```python
from build123d import *

# Parameters (mm, degrees)
F0_R     = 20
F0_R_2   = 9.5
F1_DEPTH = 50
F2_R     = 10
F3_DEPTH = 25
F5_D     = 5
F5_DEPTH = 50
F5_TIP   = 1.5021515476
F7_D     = 5
F7_DEPTH = 50
F7_TIP   = 1.5021515476
F8_R     = 1


with BuildPart() as f1:
    # F0 (on Front) → F1 (new body)
    with BuildSketch(Plane.XZ):
        Circle(F0_R)
        Circle(F0_R_2, mode=Mode.SUBTRACT)
    extrude(amount=F1_DEPTH)

    # F2 (on face) → F3 (cut)
    with BuildSketch(Plane.XZ.offset(50)):
        Circle(F2_R)
    extrude(amount=-F3_DEPTH, mode=Mode.SUBTRACT)

    # F5 (one way)
    with BuildSketch(Plane.YZ):
        with Locations((-42, 0), (-32, 0), (-18, 0), (-8, 0)):
            Circle(F5_D / 2)
    extrude(amount=-F5_DEPTH, mode=Mode.SUBTRACT)
    with Locations(Plane.YZ):
        with Locations((-42, 0), (-32, 0), (-18, 0), (-8, 0)):
            with Locations((0, 0, -(F5_DEPTH + F5_TIP / 2))):  # 118° drill point
                Cone(0, F5_D / 2, F5_TIP, mode=Mode.SUBTRACT)

    # F7 (one way)
    with BuildSketch(Plane.XY):
        with Locations((0, -8), (0, -18), (0, -32), (0, -42)):
            Circle(F7_D / 2)
    extrude(amount=-F7_DEPTH, mode=Mode.SUBTRACT)
    with Locations(Plane.XY):
        with Locations((0, -8), (0, -18), (0, -32), (0, -42)):
            with Locations((0, 0, -(F7_DEPTH + F7_TIP / 2))):  # 118° drill point
                Cone(0, F7_D / 2, F7_TIP, mode=Mode.SUBTRACT)

    # F8
    f8_edges = [f1.edges().sort_by_distance(p)[0] for p in [
        (-9.5, 0, 0),
        (-10, -50, 0),
    ]]
    fillet(f8_edges, radius=F8_R)


solid = f1.part
```
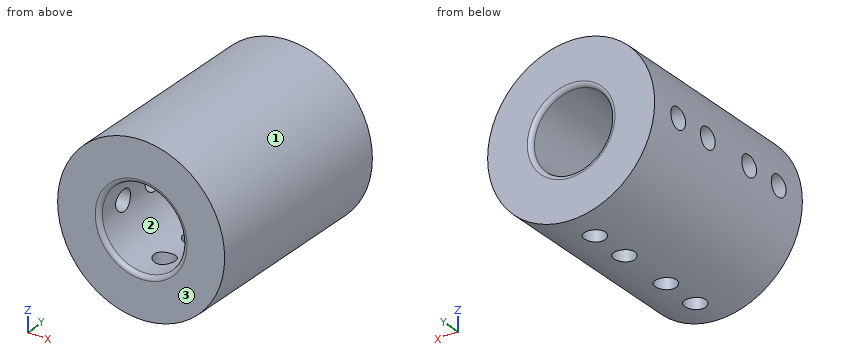
Input: part model. Units: mm. Frame: model coordinates. Face numbers are marked on the shaded views. Give positions to 0.01 mm unless a question says otherwise; leave off trailing zeros. Loops run counter-clockwise (first coordinate to the right, second up) from the corner with the lowest first, then second, coordinate; pieces in that order, holes last.
1) Section query D-D on x = -16. Return the cut outline in (y, z).
A:
outline: (-50, -12) - (0, -12) - (0, 12) - (-50, 12) - close; hole circle Ø5 at (-42, 0); hole circle Ø5 at (-32, 0); hole circle Ø5 at (-18, 0); hole circle Ø5 at (-8, 0)
2) Section query A-A on x = 0. Count the separate pieces of the cut face and the enclosed holes in it, and give its area (3 significant figures).
A:
separate pieces: 6
enclosed holes: 0
area: 819 mm2
3) Section query C-C on y = -8. Return the cut outline in (x, z).
A:
outline: (-19.84, -2.5) arc R20 ccw to (-2.5, -19.84) - (-2.5, -9.17) arc R9.5 cw to (-9.17, -2.5) - close; (-19.84, 2.5) - (-9.17, 2.5) arc R9.5 cw (long way) to (2.5, -9.17) - (2.5, -19.84) arc R20 ccw (long way) to start
4) Contact query for flat-ended pins moving along their axis: pin 1 (8 mm diameter, centred on y = -29, z = 10, fed in from -X); pin 2 (3 mm diameter, centred on y = -11.5, z = 2, fed in from +X); pin 3 (4 mm diameter, centred on x = 0, y = -32, fed in from +Z). Output: stop coordinate, or through.
A:
pin 1: stops at x = -19.08
pin 2: stops at x = 19.99
pin 3: stops at z = 20
5) Line query: L1, parallel to Y at x = 0, z = -15; L2, parallel to X at y = -38.5, z = 0; L3, parallel to Z at x = 0.5, y = -15. Output: solid intervals per line, ascending.
A:
L1: y = -50 to -44.5, -39.5 to -34.5, -29.5 to -20.5, -15.5 to -10.5, -5.5 to 0
L2: x = -20 to -10, 10 to 20
L3: z = -19.99 to -9.49, 9.49 to 19.99
6) Mould query, pull axis Z, two halves, no side actions, for the marked faces 1, 2 and 3. Classes: released by +Z, released by -Z, zero draft, split by the parting line, or undercut.
A:
face 1: split by the parting line
face 2: undercut
face 3: zero draft
